from build123d import *

# Parameters (mm, degrees)
SKETCH_1_R          = 2
EXTRUDE_1_DEPTH     = 4
FILLET_1_R          = 10
FILLET_2_R          = 2
SKETCH_8_R          = 3.300000000000001
EXTRUDE_3_DEPTH     = 5
CHAMFER_1_SIZE      = 5
SKETCH_9_R          = 3.300000000000001
CUT_EXTRUDE_3_DEPTH = 5
CHAMFER_2_SIZE      = 5


with BuildPart() as part:
    # ｽｹｯﾁ1 → ﾎﾞｽ - 押し出し1 (new body)
    # profile 1 of 5: a face of its own
    with BuildSketch(Plane.XY):
        with BuildLine():
            ThreePointArc((-27.5, 2.1540659228538024), (-27.33345237791561, 2.333452377915602), (-27.15406592285381, 2.49999999999999))
            Line((-27.154065922853814, 2.499999999999997), (-27.499999999999996, 2.499999999999997))
            Line((-27.499999999999996, 2.499999999999997), (-27.499999999999996, 2.154065922853802))
        make_face()
    # profile 2 of 5: a face of its own
    with BuildSketch(Plane.XY):
        with BuildLine():
            Line((-27.5, -2.500000000000003), (-27.154065922853817, -2.500000000000003))
            ThreePointArc((-27.154065922853817, -2.499999999999992), (-27.333452377915613, -2.3334523779156044), (-27.5, -2.1540659228538055))
            Line((-27.5, -2.1540659228538055), (-27.5, -2.500000000000003))
        make_face()
    # profile 3 of 5: a face of its own
    with BuildSketch(Plane.XY):
        with BuildLine():
            ThreePointArc((-20.10102051443362, 2.49999999999994), (-30.499999999999996, -2.39e-15), (-20.101020514433618, -2.4999999999999454))
            Line((-20.1010205144336, -2.500000000000002), (-22.84593407714621, -2.5000000000000027))
            ThreePointArc((-22.845934077146207, -2.5000000000000133), (-25.000000000000018, -3.3000000000000043), (-27.154065922853817, -2.499999999999992))
            Line((-27.154065922853817, -2.500000000000003), (-27.5, -2.500000000000003))
            Line((-27.5, -2.500000000000003), (-27.5, -2.1540659228538055))
            ThreePointArc((-27.5, -2.1540659228538055), (-28.3, -1.19e-15), (-27.5, 2.1540659228538024))
            Line((-27.499999999999996, 2.154065922853802), (-27.499999999999996, 2.499999999999997))
            Line((-27.499999999999996, 2.499999999999997), (-27.154065922853814, 2.499999999999997))
            ThreePointArc((-27.15406592285381, 2.49999999999999), (-25.000000000000014, 3.299999999999998), (-22.845934077146207, 2.500000000000007))
            Line((-22.84593407714621, 2.4999999999999982), (-20.1010205144336, 2.4999999999999987))
        make_face()
    # profile 4 of 5: a face of its own
    with BuildSketch(Plane.XY):
        with BuildLine():
            Line((-22.84593407714621, -2.5000000000000027), (-20.1010205144336, -2.500000000000002))
            ThreePointArc((-20.101020514433618, -2.4999999999999454), (-19.652365608485606, -1.2856151891963796), (-19.500000000000004, -4.41e-15))
            ThreePointArc((-19.500000000000004, -3.06e-15), (-19.652365608485606, 1.2856151891963756), (-20.10102051443362, 2.49999999999994))
            Line((-20.1010205144336, 2.4999999999999987), (-22.84593407714621, 2.4999999999999982))
            ThreePointArc((-22.845934077146207, 2.5000000000000067), (-22.00013187411367, 1.3750604449591433), (-21.7, -3.06e-15))
            ThreePointArc((-21.7, -3.87e-15), (-22.00013187411367, -1.3750604449591517), (-22.845934077146207, -2.5000000000000133))
        make_face()
    # profile 5 of 5: a face of its own
    with BuildSketch(Plane.XY):
        with BuildLine():
            Line((-20.1010205144336, -2.500000000000002), (2.5, -2.4999999999999996))
            Line((2.5, -2.4999999999999996), (2.499999999999999, 2.500000000000005))
            Line((2.499999999999999, 2.500000000000005), (-20.1010205144336, 2.4999999999999987))
            ThreePointArc((-20.10102051443362, 2.49999999999994), (-19.652365608485606, 1.2856151891963756), (-19.500000000000004, -3.06e-15))
            ThreePointArc((-19.500000000000004, -4.41e-15), (-19.652365608485606, -1.2856151891963796), (-20.101020514433618, -2.4999999999999454))
        make_face()
        Circle(SKETCH_1_R, mode=Mode.SUBTRACT)
    extrude(amount=EXTRUDE_1_DEPTH)

    # ﾌｨﾚｯﾄ1
    fillet_1_edges = [part.edges().sort_by_distance(p)[0] for p in [
        (-20.10102051443361, 2.4999999999999694, 2),
        (-20.10102051443361, -2.4999999999999742, 2),
    ]]
    fillet(fillet_1_edges, radius=FILLET_1_R)

    # ﾌｨﾚｯﾄ2
    fillet_2_edges = [part.edges().sort_by_distance(p)[0] for p in [
        (2.499999999999999, 2.500000000000005, 2),
        (2.5, -2.4999999999999996, 2),
    ]]
    fillet(fillet_2_edges, radius=FILLET_2_R)

    # ｽｹｯﾁ8 → ﾎﾞｽ - 押し出し3 (add)
    with BuildSketch(Plane(origin=(0, 0, 0), x_dir=(-1, 0, 0), z_dir=(0, 0, -1))):
        with BuildLine():
            Line((15.83484861008833, 2.5), (15.834848610088294, -2.500000000000004))
            ThreePointArc((15.834848610088294, -2.500000000000004), (18.945703694279587, -2.996180733770167), (21.747849506805537, -4.435483870967743))
            ThreePointArc((21.747849506805537, -4.435483870967743), (30.499999999999996, -3.06e-15), (21.747849506805537, 4.435483870967737))
            ThreePointArc((21.747849506805537, 4.435483870967737), (18.9457036942796, 2.996180733770169), (15.83484861008833, 2.5))
        make_face()
        with Locations((25, -3.06e-15)):
            Circle(SKETCH_8_R, mode=Mode.SUBTRACT)
    extrude(amount=EXTRUDE_3_DEPTH)

    # 面取り1
    chamfer_1_edges = [part.edges().sort_by_distance(p)[0] for p in [
        (-15.834848610088311, -1.78e-15, 0),
    ]]
    chamfer(chamfer_1_edges, length=CHAMFER_1_SIZE - 0.0001)  # a hair under: the kernel refuses the full size

    # ｽｹｯﾁ9 → ｶｯﾄ - 押し出し3 (cut)
    with BuildSketch(Plane.XY.offset(4)):
        with BuildLine():
            Line((-18.834848610088333, -2.960607985830548), (-18.83484861008833, 2.9606079858305425))
            ThreePointArc((-18.83484861008833, 2.9606079858305425), (-20.351950663989726, 3.5783527846792875), (-21.747849506805537, 4.435483870967737))
            ThreePointArc((-21.747849506805537, 4.435483870967737), (-30.499999999999996, -1.29e-15), (-21.747849506805537, -4.435483870967743))
            ThreePointArc((-21.747849506805537, -4.435483870967743), (-20.35195066398973, -3.5783527846792946), (-18.834848610088333, -2.960607985830548))
        make_face()
        with Locations(Location((-25, -3.06e-15, 0), (0, 0, 180))):
            Circle(SKETCH_9_R, mode=Mode.SUBTRACT)
    extrude(amount=-CUT_EXTRUDE_3_DEPTH, mode=Mode.SUBTRACT)

    # 面取り2
    chamfer_2_edges = [part.edges().sort_by_distance(p)[0] for p in [
        (-18.83484861008833, -2.66e-15, 4),
    ]]
    chamfer(chamfer_2_edges, length=CHAMFER_2_SIZE - 0.0001)  # a hair under: the kernel refuses the full size


solid = part.part
For this review, take the finished solid that the model builds, in its own axes (mm). A direction names the side the tool comes from. Round coordinates to 2 decimals unless told otherwise and drop trailing zeros. Write each loop counter-clockwise with the first axis right and the second up, starting at its lowest first coordinate (ties: lowest second). Pieces come first, ordered by that corner, then holes. Notation, with made-up numbers: (37.25, 19) -> (84.25, 19) arc R32 ccw to (84.25, 51) -> close; hole circle Ø5 at (45, 32). An arc over 180 degrees is marked (long way). Use CSV: the item, a comma, the result in double quotes.
(1) Consider section B-B, the plane y = 0. Give the number of separate pieces and of enclosed holes in the cut face, plus the area to 3 significant figures.
Computed values:
separate pieces,"3"
enclosed holes,"0"
area,"105 mm²"
(2) Consider section C-C, the plane z = -4. Give the boundary of the cut face in (x, y), plus the area to 3 significant figures.
Computed values:
outline,"(-21.75, -4.44) arc R10 cw to (-15.83, -2.5) -> (-14.83, -2.5) -> (-14.83, 2.5) -> (-15.83, 2.5) arc R10 cw to (-21.75, 4.44) arc R5.5 ccw (long way) to start; hole circle Ø6.6 at (-25, 0)"
area,"88.7 mm²"
(3) Clearance check with flat-ended pins moving along their axes: P1, Ø2, axis at x = -11, z = 2, coming from the +Y side; P2, Ø5.5, axis at x = -23.5, y = 1, coming from the +Z side; P3, Ø4, axis at x = -3.5, y = 0, coming from the -Z side; P4, Ø3.5, axis at x = 0, y = 0, coming from the +Z side. State where each tip first meets the part, or that it passes through.
Computed values:
P1,"y = 2.5"
P2,"z = -1"
P3,"z = 0"
P4,"through"
(4) To check wall thickness, follow L1, parallel to Y at x = 0, z = 1.8; L2, parallel to Y at x = -25, z = -2.95; L3, parallel to Y at x = -13, z = -1.75. State the ranges of each line that lie inside material, in increasing order. Write a range as [from, to].
Computed values:
L1,"[-2.5, -2], [2, 2.5]"
L2,"[-5.5, -3.3], [3.3, 5.5]"
L3,"[-2.5, 2.5]"
(5) Draft analysis for pull direction X (two halves, no side actions). For faces 1 (the face through (-13.3, 0.035, -2.465)), 2 (the face through (-28.15, 0.99, -2.97)), 3 (the face through (-8, 2.5, 1)), state which applies: +X half, -X half, draft (parallel to the pull), parting line (faces both ways), or undercut.
Computed values:
face 1,"+X half"
face 2,"undercut"
face 3,"draft"
(6) For faces 4 (the face through (-6, 0, 0)), 5 (the face through (-8, -2.5, 1)), 6 (the face through (-22, -2, -1)), list the 3-axis set-ups (+Z, -Z, +X, -X, +Y, -Y) from which the entire face can be reached by the end or side of a thin tool; tool diameter is ignored.
Computed values:
face 4,"-Z, +X, +Y, -Y"
face 5,"+Z, -Z, +X, -Y"
face 6,"+Z, -X, +Y, -Y"
(7) Consider section A-A, the plane x = -25. Give the boundary of the cut face in (y, z), plus the area to 3 significant figures.
Computed values:
outline,"(-5.5, -5) -> (-3.3, -5) -> (-3.3, -1) -> (-5.5, -1) -> close; (3.3, -5) -> (5.5, -5) -> (5.5, -1) -> (3.3, -1) -> close"
area,"17.6 mm²"
(8) Consider section D-D, the plane x = 0. Give the boundary of the cut face in (y, z), plus the area to 3 significant figures.
Computed values:
outline,"(-2.5, 0) -> (-2, 0) -> (-2, 4) -> (-2.5, 4) -> close; (2, 0) -> (2.5, 0) -> (2.5, 4) -> (2, 4) -> close"
area,"4.00 mm²"
